Geometry: see drawing. Coordinates: mm, zero at the bounding-box minimum. A direction names the side the tool comes from. Give positions to 0.01 mm unless a question says otherwise; leave off trailing zeros. Order: outer loops, then holes, each group sorted by start corner. A loop starts at its lowest first (then second) coordinate and runs counter-clockwise, first axis right, second up. Notation, with made-up numbers: M 74,-9 L 94,-9 A13 cw 94,2 Z; hole C -13,-4 d4. An arc over 180 degrees is marked long. Use a Markdown table: item, result.
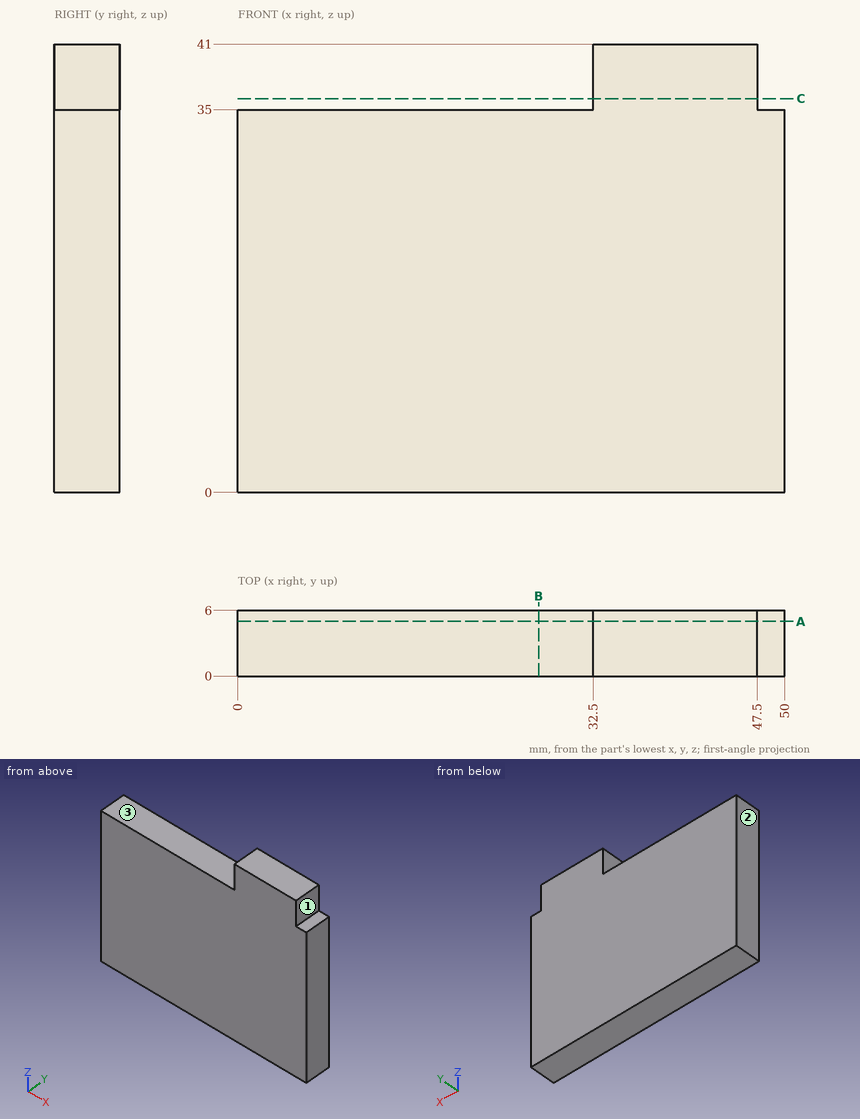
1) Cut plane A-A on y = 5. Return loops of the section in (x, z).
Response values:
| item | result |
|---|---|
| outline | M 0,0 L 50,0 L 50,35 L 47.5,35 L 47.5,41 L 32.5,41 L 32.5,35 L 0,35 Z |
2) Cut plane B-B on x = 27.5. Return loops of the section in (y, z), and give its area (3 significant figures).
Response values:
| item | result |
|---|---|
| outline | M 0,0 L 6,0 L 6,35 L 0,35 Z |
| area | 210 mm² |
3) First-contact query: pin 1 Ø0.8 at (x, y) = (48.5, 3.5) entering from +Z; pin 2 Ø3 at (y, z) = (3, 38) entering from -X. Flat tips, straight axial feed; report the tip coordinate or a pass-through.
Response values:
| item | result |
|---|---|
| pin 1 | stops at z = 35 |
| pin 2 | stops at x = 32.5 |
4) Cut plane C-C on z = 36. Return loops of the section in (x, y).
Response values:
| item | result |
|---|---|
| outline | M 32.5,0 L 47.5,0 L 47.5,6 L 32.5,6 Z |
5) Reachability of the marked faces 1, 2 and 3 from +Z, -Z, +X, -X, +Y, -Y: full face, straight path, thin tool, end or side. Return the list, or none.
Response values:
| item | result |
|---|---|
| face 1 | +Z, +X, +Y, -Y |
| face 2 | +Z, -Z, -X, +Y, -Y |
| face 3 | +Z, -X, +Y, -Y |
6) Material intervals for line 1 (X direction, y = 3.2, z = 38); line 2 (Z direction, x = 8, y = 3.05), sorted ascending. Write a range as from..to.
Response values:
| item | result |
|---|---|
| line 1 | x = 32.5..47.5 |
| line 2 | z = 0..35 |
